Could you check a few things on this model? Use its own coordinates, in mm. Coordinates: 2 decimals unless noted, no trailing zeros. Order: outer loops, then holes, each group sorted by start corner. A loop starts at its lowest first (then second) coordinate and runs counter-clockwise, first axis right, second up. Notation, with made-up numbers: (-33, 14) - (4, 14) arc R11 cw to (4, 30) - close; hole circle Ø9 at (-19, 14). An arc over 180 degrees is marked (long way). One line per item, written item: value.
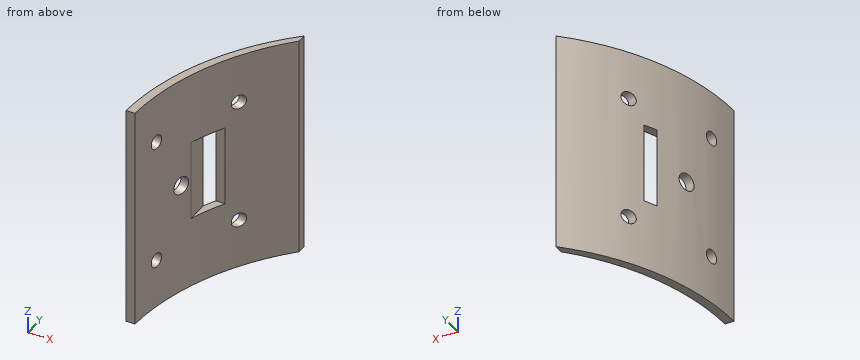
Autodesk Inventor part; units mm, degrees
ref_plane "Work Plane1" through (0, 0, 62.5) normal (0, 0, -1) x (-1, 0, 0)
ref_plane "Work Plane2" through (-10, 0, 62.5) normal (-0.9866, 0.1632, 0) x (-0.1632, -0.9866, 0)
ref_plane "YZ Plane" through (0, 0, 0) normal (1, 0, 0) x (0, 1, 0)
sketch "Sketch1" plane through (0, 0, 0) normal (0, 0, 1) x (1, 0, 0)
  arc A0 (45, 98) -> (0, 0) centre (139.9137, -4.9145) ccw
  line L0 (45, 98) -> (45, 93)
  line L1 (0, 0) -> (5, 0)
  arc A1 (45, 93) -> (5, 0) centre (144.908, -5.0734) ccw
  dimension "d0" = 140
  dimension "d1" = 98
  dimension "d3" = 45
  dimension "d4" = 5
  dimension "d5" = 5
  dimension "d6" = 140
extrude "Extrusion1" add sketch "Sketch1" along normal blind 125
ref_plane "Work Plane1" through (0, 0, 62.5) normal (0, 0, -1) x (-1, 0, 0)
ref_plane "Work Plane2" through (-10, 0, 62.5) normal (-0.9866, 0.1632, 0) x (-0.1632, -0.9866, 0)
sketch "Sketch2" plane through (-10, 0, 62.5) normal (-0.9866, 0.1632, 0) x (-0.1632, -0.9866, 0)
  circle A0 centre (-20.6619, -35) radius 4
  circle A1 centre (-72.6619, -35) radius 4
  circle A2 centre (-20.6619, 35) radius 4
  circle A3 centre (-72.6619, 35) radius 4
  line L0 (0, 42.5) -> (0, -42.5)
  line L1 (-72.6619, 35) -> (-20.6619, 35) construction
  line L2 (-20.6619, 35) -> (-20.6619, -35) construction
  line L3 (-20.6619, -35) -> (-72.6619, -35) construction
  line L4 (-72.6619, -35) -> (-72.6619, 35) construction
  line L5 (-105.6619, -42.5) -> (-105.6619, 42.5)
  point P0 (0, 0)
  point P1 (-20.6619, 0)
  point P2 (0, 0)
  dimension "d9" = 8
  dimension "d10" = 8
  dimension "d12" = 52
  dimension "d14" = 8
  dimension "d15" = 8
  dimension "d16" = 70
  dimension "d23" = 33
extrude "Extrusion2" cut sketch "Sketch2" against normal through all
sketch "Sketch4" plane through (-10, 0, 62.5) normal (-0.9866, 0.1632, 0) x (-0.1632, -0.9866, 0)
  circle A0 centre (-38.6319, 0) radius 5
  line L0 (-1.6319, 62.5) -> (-1.6319, -62.5)
  point P0 (-1.6319, 0)
  dimension "d24" = 10
  dimension "d25" = 37
extrude "Extrusion4" cut sketch "Sketch4" against normal through all
sketch "Sketch5" plane through (45, 93, 0) normal (1, 0, 0) x (0, 0, -1)
  line L0 (-40, -32) -> (-85, -32)
  line L1 (-85, -32) -> (-85, -93)
  line L2 (-85, -93) -> (-40, -93)
  line L3 (-40, -93) -> (-40, -32)
  line L4 (0, -93) -> (-125, -93)
  line L5 (0, 0) -> (-125, 0)
  point P0 (-62.5, -32)
  point P1 (-62.5, -93)
  point P2 (-62.5, -93)
  dimension "d28" = 45
  dimension "d31" = 32
extrude "Extrusion5" cut sketch "Sketch5" against normal blind 32
properties part number "SJ009" material "ABS Plastic"
Item 1: I want a section at A-A on z = 47.5. Please give me the cut outline in (x, y), then the cut area to 3 significant figures.
Conclusion:
outline: (0, 0) - (5, 0) arc R140 cw to (13, 41.83) - (13, 54.19) arc R140 ccw to start; (16.4, 61) - (21.48, 61) arc R140 cw to (45, 93) - (45, 98) arc R140 ccw to start
area: 419 mm²
Item 2: I want a section at B-B on y = 57. Please give me the cut outline in (x, z).
Conclusion:
outline: (14.35, 0) - (19.42, 0) - (19.42, 40) - (14.35, 40) - close; (14.35, 85) - (19.42, 85) - (19.42, 125) - (14.35, 125) - close
Item 3: If I drill on probe 1 along Z at (x, y) = (24, 69); probe 2 along Y at (x, z) = (38.5, 20); probe 3 along Y at (x, z) = (43.5, 42.5), over which ranges is the centre line in solid material (lowest first)?
Conclusion:
probe 1: 0 to 23.62, 31.38 to 93.62, 101.38 to 125
probe 2: 85.91 to 91.6
probe 3: 91.45 to 96.6
Item 4: I want a section at D-D on y = 16.5. Give the number of separate pieces and of enclosed holes in the cut face, then the cut area to 3 significant figures.
Conclusion:
separate pieces: 3
enclosed holes: 0
area: 559 mm²
Item 5: I want a section at C-C on z = 19. Please give me the cut outline in (x, y), then the cut area to 3 significant figures.
Conclusion:
outline: (0, 0) - (5, 0) arc R140 cw to (45, 93) - (45, 98) arc R140 ccw to start
area: 484 mm²
Item 6: I'm going to push flat-ended pins straight in: pin 1 Ø12 at (x, y) = (5, 14.5) entering from -Z; pin 2 Ø2 at (x, z) = (29, 21) entering from -Y; pin 3 Ø8 at (x, y) = (14.5, 28.5) entering from +Z; pin 4 Ø2.5 at (x, z) = (20, 54) entering from -Y. Where does each tip first touch, or does it pass through?
Conclusion:
pin 1: z = 0
pin 2: y = 71.95
pin 3: through
pin 4: y = 61
